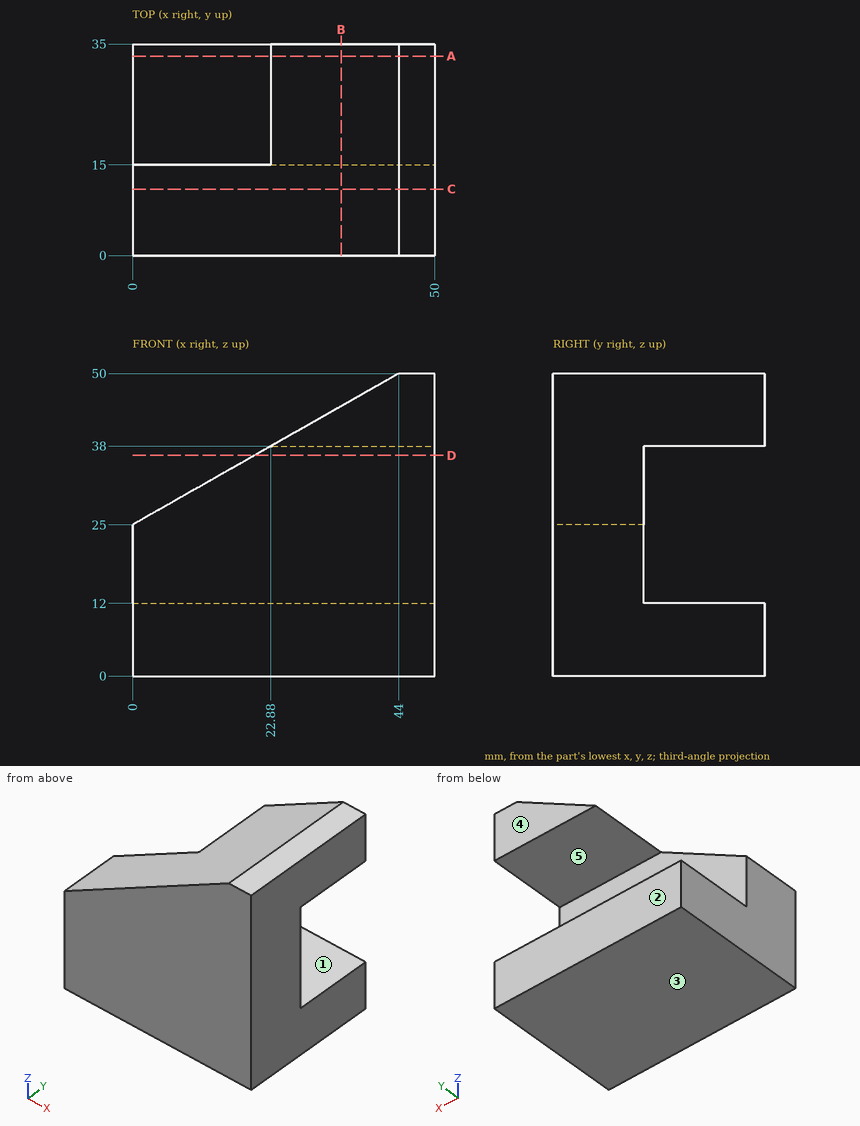
Could you check a few things on this drawing? It's one solid part, dimensions in mm from its lowest x, y, z. A direction names the side the tool comes from. Coordinates: 2 decimals unless noted, no trailing zeros. Order: outer loops, then holes, each group sorted by start corner. A loop starts at its lowest first (then second) coordinate and runs counter-clockwise, first axis right, second up. Notation, with made-up numbers: (-24.75, 44) - (31.25, 44) arc R32 cw to (31.25, 71) - close; hole circle Ø1 at (6, -5). An arc over 180 degrees is marked (long way). Answer as a JSON object with one key per item and string values. Group by question number.
Q1. We'd pull the mould along Z, two halves only. Please class the marked faces 1, 2 and 3: +Z half, -Z half, draft (parallel to the pull), parting line (faces both ways), or undercut.
Q2. Will these pins go through, and if not, where does the flat tip stop? P1, Ø3, axis at x = 24.5, y = 25, coming from the +Z side; P2, Ø6, axis at x = 37, y = 26, coming from the +Z side; P3, Ø4, axis at y = 8, z = 22.5, coming from the -X side; P4, Ø8, axis at x = 23.5, z = 31.5, coming from the +Y side.
Q3. Imagine slicing it at C-C (y = 11). Please give me the cut outline in (x, z), and give its area (3 significant figures).
Q4. I need wall thicknesses on line 1 (Y direction, x = 13, z = 29.5); line 2 (Z direction, x = 31, y = 20.5); line 3 (Z direction, x = 27.5, y = 28) (3 decimals). Which ranges of each line are inside material? Lowest first, please. Write a range as from..to.
Q5. Imagine slicing it at B-B (x = 34.5). Please give me the cut outline in (y, z), and give its area (3 significant figures).
Q6. Imagine slicing it at D-D (z = 36.5). Please give me the cut outline in (x, y), and give its area (3 significant figures).
Q7. On a 3-axis mill with a long thin cutter (end or side, diameter ignored), from which of +Z, -Z, +X, -X, +Y, -Y can I reach the whole of each face in a straight line? I mean the marked faces 4 and 5. Say none if no direction works.
Q8. Imagine slicing it at A-A (y = 33). Please give me the cut outline in (x, z), and give its area (3 significant figures).
Determined:
{
 "1": {"face 1": "undercut", "face 2": "draft", "face 3": "-Z half"},
 "2": {"P1": "stops at z = 39.77", "P2": "stops at z = 47.73", "P3": "stops at x = 0", "P4": "stops at y = 15"},
 "3": {"outline": "(0, 0) - (50, 0) - (50, 50) - (44, 50) - (0, 25) - close", "area": "1,950 mm2"},
 "4": {"line 1": "y = 0..15", "line 2": "z = 0..12, 38..42.61", "line 3": "z = 0..12, 38..40.625"},
 "5": {"outline": "(0, 0) - (35, 0) - (35, 12) - (15, 12) - (15, 38) - (35, 38) - (35, 44.6) - (0, 44.6) - close", "area": "1,040 mm2"},
 "6": {"outline": "(20.24, 0) - (50, 0) - (50, 15) - (20.24, 15) - close", "area": "446 mm2"},
 "7": {"face 4": "+Z, -Z, +X, -X, +Y", "face 5": "+X, -X, +Y"},
 "8": {"outline": "(0, 0) - (50, 0) - (50, 12) - (0, 12) - close; (22.88, 38) - (50, 38) - (50, 50) - (44, 50) - close", "area": "799 mm2"}
}
